Check sheet for the modelled part. Datum: model origin and axes. Units: mm. Face numbers are marked on the shaded views. A direction names the side the tool comes from. Coordinates: 2 decimals unless noted, no trailing zeros. Order: outer loops, then holes, each group sorted by start corner. A loop starts at its lowest first (then second) coordinate and runs counter-clockwise, first axis right, second up.
1. Cross-section at C-C (y = 338.5). Enter the section's corners in (x, z), then the cut area to 3 significant figures.
2. Draft check along Z on the marked faces 3, 4 and 5. Enter one of: released by +Z, released by -Z, zero draft, split by the parting line, or undercut.
3. Cross-section at B-B (z = 0). Enter the section's corners in (x, y).
4. Gauge pin test, flat ends, axial feed: pin 1 Ø4 at (y, z) = (117, -77.5) entering from -X; pin 2 Ø6 at (y, z) = (328, 143) entering from -X; pin 3 Ø5 at (x, z) = (-137.5, 128.5) entering from +Y. Record the tip position at first contact, or that the pin passes through.
5. Cross-section at A-A (x = 0). Enter the section's corners in (y, z), then the cut area to 3 significant figures.
6. Thickness scan on line 1 (X direction, y = 207, z = 0); line 2 (Y direction, x = 15.5, z = 57.5). Record the ranges inside material, lowest first.
7. Cross-section at D-D (y = -15). Enter the section's corners in (x, z), then the cut area to 3 significant figures.
8. Set-up check for the marked faces 1 and 2: record each of +Z, -Z, +X, -X, +Y, -Y from which the full face is reachable in a straight line by a thin tool's end or side.
```python
from build123d import *

# Parameters (mm, degrees)
SKETCH_1_R        = 175
SKETCH_1_R_2      = 170
EXTRUDE_1_DEPTH   = 400
EXTRUDE_1_2_DEPTH = 50


with BuildPart() as part:
    # Эскиз1 → Extrude 1 (new body)
    with BuildSketch(Plane(origin=(0, 0, 0), x_dir=(1, 0, 0), z_dir=(0, 1, 0))):
        Circle(SKETCH_1_R)
        Circle(SKETCH_1_R_2, mode=Mode.SUBTRACT)
    extrude(amount=EXTRUDE_1_DEPTH)

    # Эскиз2 → Extrude 1 2 (add)
    with BuildSketch(Plane.XZ):
        with BuildLine():
            Line((-64.674331545, -230), (64.667769704, -230))
            ThreePointArc((64.667769704, -230), (78.320322733, -226.713438487), (88.981545406, -217.573853052))
            Line((88.981545406, -217.573853052), (169.425013579, -106.278712703))
            ThreePointArc((169.425013579, -106.278712703), (-0.414705995, 199.999570047), (-168.982813438, -106.980412985))
            Line((-168.982813438, -106.980412985), (-88.982009615, -217.582286166))
            ThreePointArc((-88.982009615, -217.582286166), (-78.322251075, -226.715806042), (-64.674331545, -230))
        make_face()
    extrude(amount=EXTRUDE_1_2_DEPTH)


solid = part.part
```
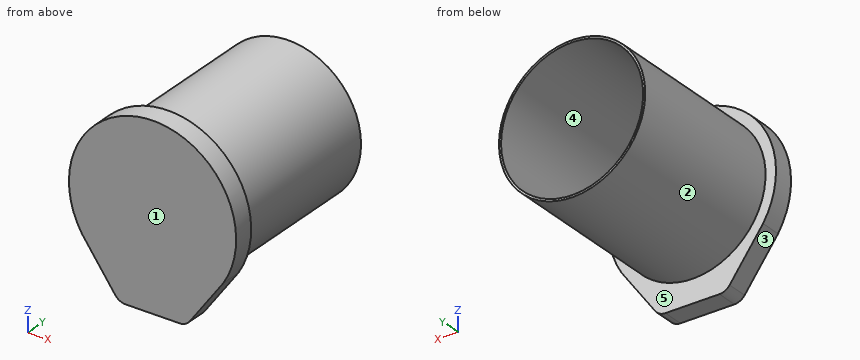
Data:
1. outline: circle Ø350 at (0, 0); hole circle Ø340 at (0, 0)
1. area: 5,420 mm2
2. face 3: released by -Z
2. face 4: undercut
2. face 5: zero draft
3. outline: (-200, -50) - (200, -50) - (200, 0) - (175, 0) - (175, 400) - (170, 400) - (170, 0) - (-170, 0) - (-170, 400) - (-175, 400) - (-175, 0) - (-200, 0) - close
4. pin 1: stops at x = -157.88
4. pin 2: stops at x = -105
4. pin 3: stops at y = 0
5. outline: (-50, -230) - (0, -230) - (0, -175) - (400, -175) - (400, -170) - (0, -170) - (0, 170) - (400, 170) - (400, 175) - (0, 175) - (0, 200) - (-50, 200) - close
5. area: 25,500 mm2
6. line 1: x = -175 to -170, 170 to 175
6. line 2: y = -50 to 0
7. outline: (-168.98, -106.98) - (-88.98, -217.58) arc R30 ccw to (-64.67, -230) - (64.67, -230) arc R30 ccw to (88.98, -217.57) - (169.43, -106.28) arc R200 ccw (long way) to start
7. area: 134,000 mm2
8. face 1: +Z, -Z, +X, -X, -Y
8. face 2: +Y
